Study the drawing (mm; zero at the part's minimum x, y, z) and answer. Round coordinates to 2 decimals unless told otherwise and drop trailing zeros. Order: outer loops, then holes, each group sorted by start corner. A loop starts at its lowest first (then second) coordinate and runs counter-clockwise, first axis right, second up. Notation, with made-up numbers: (26, 30.25) - (83, 30.25) arc R17 ccw to (83, 37.25) - close; hole circle Ø8 at (35, -27.5). An arc over 180 degrees is marked (long way). Put each result on its own line as item: value. Start each with the question number.
Q1. Each of these flat-tipped pins is pushed along its axis until it touches: pin 1 Ø1 at (y, z) = (3.5, 111.5) entering from +X; pin 2 Ø20.5 at (x, z) = (127, 234.95) entering from +Y; pin 3 Ø1.5 at (y, z) = (5.5, 181) entering from -X; pin 4 Ø2 at (y, z) = (3.5, 208) entering from -X (1 decimal). Where does it stop, or does it pass through?
Q2. Section C-C on y = 1 is taken. State how many separate pieces and enclosed holes the cut face has, then the cut area to 3 significant figures.
Q3. Find the intervals of material crossed by line 1 along X through (y, z) = (1.5, 182) (1 decimal); line 2 along X through (y, z) = (1.75, 127); line 3 along X through (y, z) = (2, 19.05) (1 decimal), in increasing order. Write a range as from..to.
Q4. Section B-B on x = 127 is taken. Give the vertices of the cut face in (y, z).
Q5. Section A-A on z = 127 is taken. Give the vertices of the cut face in (x, y).
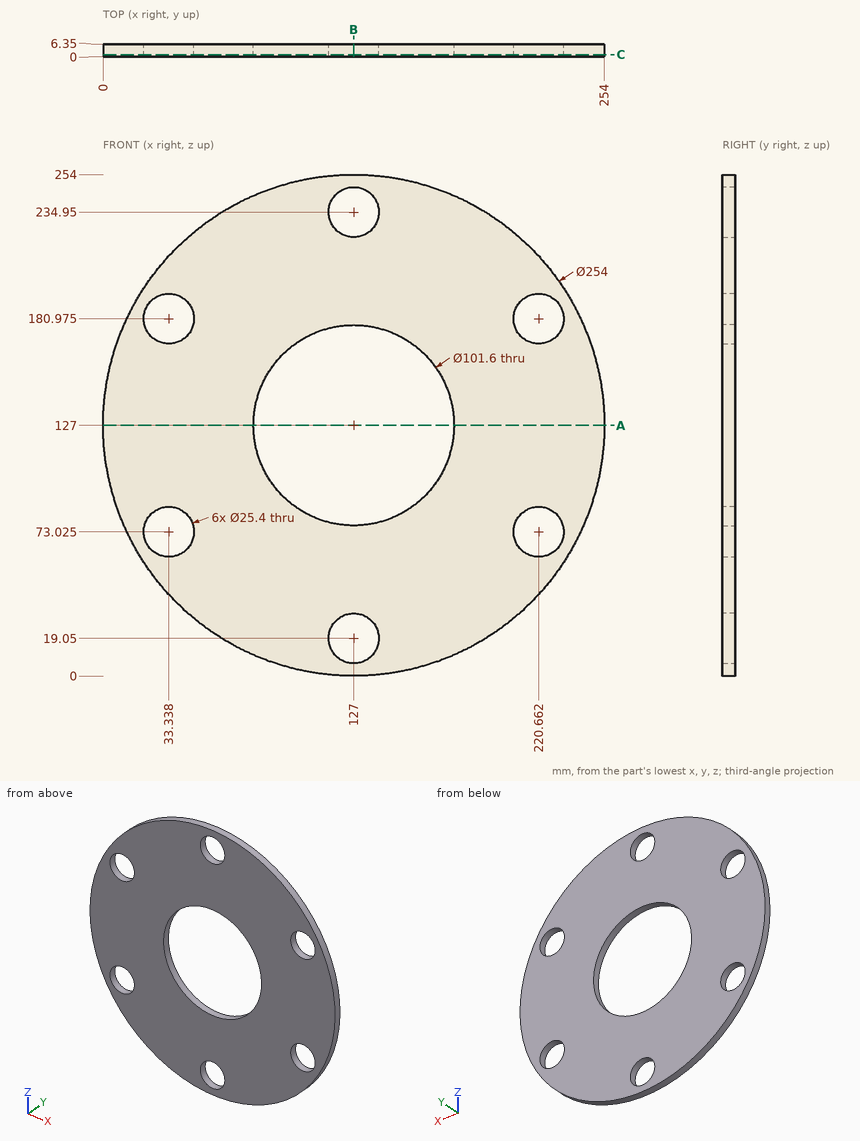
Findings:
1. pin 1: x = 253.11
1. pin 2: through
1. pin 3: x = 11.7
1. pin 4: x = 28.4
2. separate pieces: 1
2. enclosed holes: 7
2. area: 39,500 mm2
3. line 1: 12.5..20.7, 46..208, 233.3..241.5
3. line 2: 0..76.2, 177.8..254
3. line 3: 60.1..114.3, 139.7..193.9
4. outline: (0, 0) - (6.35, 0) - (6.35, 6.35) - (0, 6.35) - close; (0, 31.75) - (6.35, 31.75) - (6.35, 76.2) - (0, 76.2) - close; (0, 177.8) - (6.35, 177.8) - (6.35, 222.25) - (0, 222.25) - close; (0, 247.65) - (6.35, 247.65) - (6.35, 254) - (0, 254) - close
5. outline: (0, 0) - (76.2, 0) - (76.2, 6.35) - (0, 6.35) - close; (177.8, 0) - (254, 0) - (254, 6.35) - (177.8, 6.35) - close
